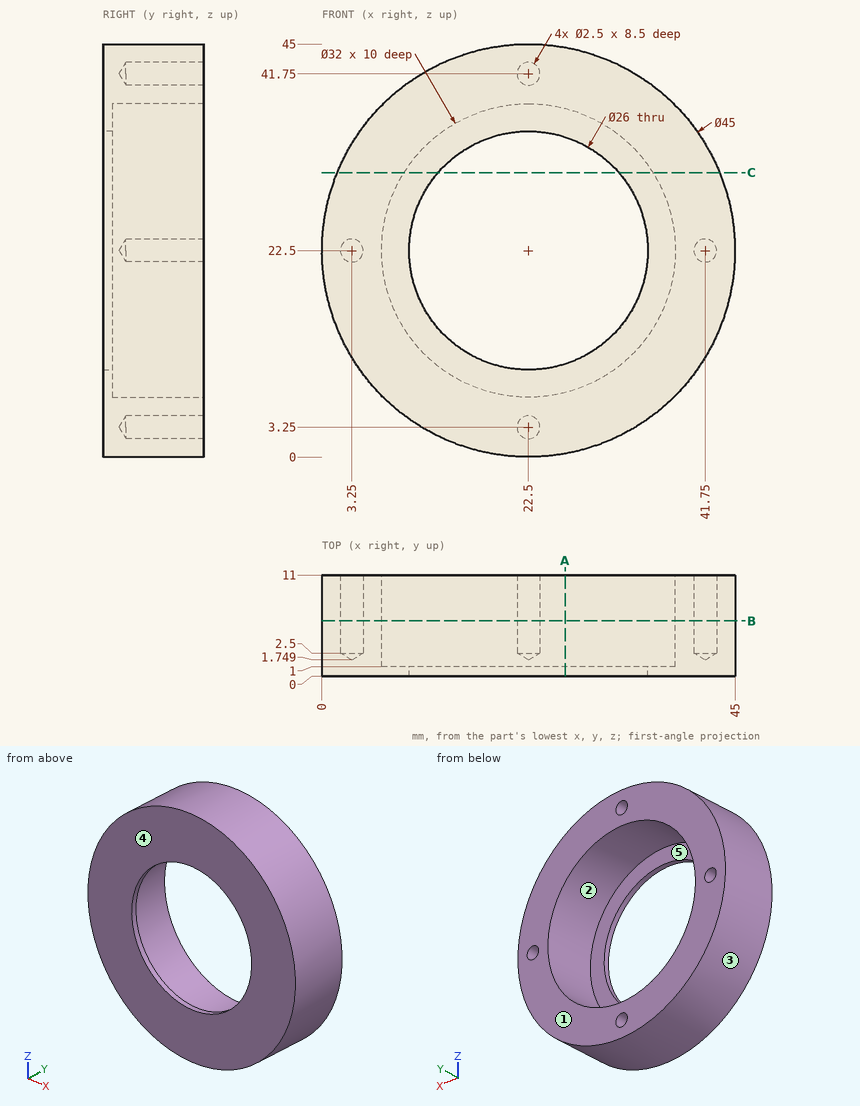
Geometry: see drawing. Coordinates: mm, zero at the bounding-box minimum. A direction names the side the tool comes from. Round coordinates to 2 decimals unless told otherwise and drop trailing zeros. Loops run counter-clockwise (first coordinate to the right, second up) from the corner with the lowest first, then second, coordinate; pieces in that order, holes last. Notation, with made-up numbers: (80.25, 34.25) -> (123.25, 34.25) arc R20 cw to (123.25, 55.25) -> close; hole circle Ø1 at (23, 2). An arc over 180 degrees is marked (long way). Use one line per item in the form item = value. Start each with the question number.
Item 1: Section query B-B on y = 6. Return the cut outline in (x, z).
Item 2: Section query C-C on z = 31. Return the cut outline in (x, y).
Item 3: Material intervals for L1, parallel to X at y = 4, z = 22.5; L2, parallel to X at y = 0.4, z = 22.5; L3, parallel to Y at x = 31.5, z = 12.5, sorted ascending. Write a range as from..to.
Item 4: Section query A-A on x = 26.5. Return the cut outline in (y, z).
Item 5: Set-up query: the marked faces 4 and 5. Return all of +Z, -Z, +X, -X, +Y, -Y with unobstructed straight access to the full face (end or side cutting, diameter ignored); none if empty.
Item 6: Mould query, pull axis Z, two halves, no side actions, for the marked faces 1, 2 and 3. Classes: pulls with the +Z half, pulls with the -Z half, needs draft (parallel to the pull), parting line crosses it, or undercut.
Item 7: Contact query for flat-ended pins moving along their axis: pin 1 Ø2 at (x, z) = (3.25, 22.5) entering from +Y; pin 2 Ø3 at (x, y) = (10, 2) entering from -Z; pin 3 Ø6 at (y, z) = (4, 37.5) entering from +X. Output: stop coordinate, or through.
Ans:
q1.outline = circle Ø45 at (22.5, 22.5); hole circle Ø2.5 at (3.25, 22.5); hole circle Ø32 at (22.5, 22.5); hole circle Ø2.5 at (22.5, 3.25); hole circle Ø2.5 at (22.5, 41.75); hole circle Ø2.5 at (41.75, 22.5)
q2.outline = (1.67, 0) -> (12.66, 0) -> (12.66, 1) -> (8.94, 1) -> (8.94, 11) -> (1.67, 11) -> close; (32.34, 0) -> (43.33, 0) -> (43.33, 11) -> (36.06, 11) -> (36.06, 1) -> (32.34, 1) -> close
q3.L1 = 0..2, 4.5..6.5, 38.5..40.5, 43..45
q3.L2 = 0..9.5, 35.5..45
q3.L3 = 0..1
q4.outline = (0, 0.36) -> (11, 0.36) -> (11, 7.01) -> (1, 7.01) -> (1, 10.13) -> (0, 10.13) -> close; (0, 34.87) -> (1, 34.87) -> (1, 37.99) -> (11, 37.99) -> (11, 44.64) -> (0, 44.64) -> close
q5.face_4 = +Z, -Z, +X, -X, -Y
q5.face_5 = +Y
q6.face_1 = needs draft
q6.face_2 = undercut
q6.face_3 = parting line crosses it
q7.pin_1 = 2.35
q7.pin_2 = 2.87
q7.pin_3 = 41.53
